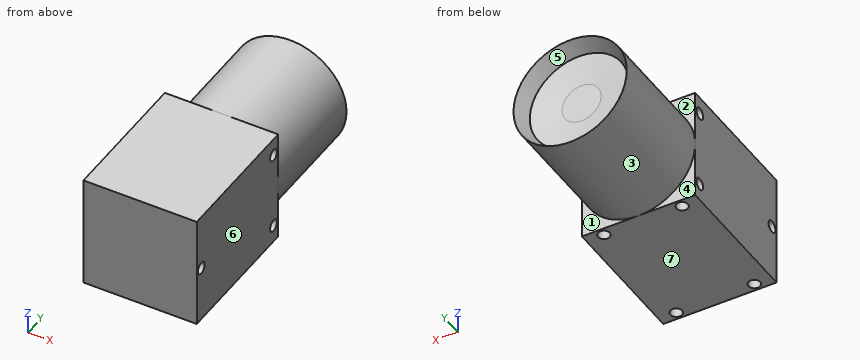
```python
from build123d import *

# Parameters (mm, degrees)
SKETCH_2_W          = 29
SKETCH_2_H          = 29
EXTRUDE_1_DEPTH     = 35.7
SKETCH_3_R          = 1.5
CUT_EXTRUDE_1_DEPTH = 4
CUT_EXTRUDE_2_REACH = 50.226
SKETCH_4_R          = 1.5


with BuildPart() as part:
    # 草图1 → 旋转1 (revolve)
    with BuildSketch(Plane.XY):
        Polygon((0, 0), (-14.5, 0), (-14.5, 30), (-12.646873789, 26.018036841), (-5, 25), (0, 25), align=None)
    revolve(axis=Axis((0, 25, 0), (0, -1, 0)))

    # 草图2 → 凸台-拉伸1 (add)
    with BuildSketch(Plane.XZ):
        Rectangle(SKETCH_2_W, SKETCH_2_H)
    extrude(amount=EXTRUDE_1_DEPTH)

    # 草图3 → 切除-拉伸1 (cut)
    with BuildSketch(Plane(origin=(0, 0, -14.5), x_dir=(-1, 0, 0), z_dir=(0, 0, -1))):
        with Locations((-10, -2)):
            Circle(SKETCH_3_R)
        with Locations((-10, -33.7)):
            Circle(SKETCH_3_R)
        with Locations(Location((10, -33.7, 0), (0, 0, 180))):
            Circle(SKETCH_3_R)
        with Locations(Location((10, -2, 0), (0, 0, 180))):
            Circle(SKETCH_3_R)
    extrude(amount=-CUT_EXTRUDE_1_DEPTH, mode=Mode.SUBTRACT)

    # 草图4 → 切除-拉伸2 (cut, up to next)
    with BuildSketch(Plane(origin=(14.5, 0, 0), x_dir=(0, 0, -1), z_dir=(1, 0, 0)), mode=Mode.PRIVATE) as cut_extrude_2_sk1:
        with Locations(Location((-10, -2, 0), (0, 0, 90))):
            Circle(SKETCH_4_R)
    cut_extrude_2_tool1 = extrude(cut_extrude_2_sk1.sketch, amount=-CUT_EXTRUDE_2_REACH, mode=Mode.PRIVATE) & part.part
    # 草图4 → 切除-拉伸2 (cut, up to next)
    with BuildSketch(Plane(origin=(14.5, 0, 0), x_dir=(0, 0, -1), z_dir=(1, 0, 0)), mode=Mode.PRIVATE) as cut_extrude_2_sk2:
        with Locations(Location((0, -33.7, 0), (0, 0, 90))):
            Circle(SKETCH_4_R)
    cut_extrude_2_tool2 = extrude(cut_extrude_2_sk2.sketch, amount=-CUT_EXTRUDE_2_REACH, mode=Mode.PRIVATE) & part.part
    # 草图4 → 切除-拉伸2 (cut, up to next)
    with BuildSketch(Plane(origin=(14.5, 0, 0), x_dir=(0, 0, -1), z_dir=(1, 0, 0)), mode=Mode.PRIVATE) as cut_extrude_2_sk3:
        with Locations(Location((10, -2, 0), (0, 0, 90))):
            Circle(SKETCH_4_R)
    cut_extrude_2_tool3 = extrude(cut_extrude_2_sk3.sketch, amount=-CUT_EXTRUDE_2_REACH, mode=Mode.PRIVATE) & part.part
    add(cut_extrude_2_tool1.solids().sort_by_distance((14.5, -2, 10))[0], mode=Mode.SUBTRACT)
    add(cut_extrude_2_tool2.solids().sort_by_distance((14.5, -33.7, 0))[0], mode=Mode.SUBTRACT)
    add(cut_extrude_2_tool3.solids().sort_by_distance((14.5, -2, -10))[0], mode=Mode.SUBTRACT)


solid = part.part
```
The listing builds one solid part. Answer for the finished solid, in the listing's coordinates (mm). Face numbers are marked on the shaded views. A direction names the side the tool comes from. Coordinates: 2 decimals unless noted, no trailing zeros. Loops run counter-clockwise (first coordinate to the right, second up) from the corner with the lowest first, then second, coordinate; pieces in that order, holes last. Notation, with made-up numbers: (-22.75, -25) -> (-12.75, -25) arc R8 cw to (-12.75, -11) -> close; hole circle Ø11 at (-15.75, 27). An arc over 180 degrees is marked (long way). Use one line per item in the form item = value. Start each with the question number.
Item 1: Flat-ended cylindrical pins translate along their axes: pin 1 Ø5 at (x, z) = (1, -2) entering from +Y; pin 2 Ø2.5 at (y, z) = (-2, 10) entering from -X; pin 3 Ø11.5 at (x, z) = (5.5, -4) entering from +Y; pin 4 Ø2.5 at (x, y) = (-10, -33.7) entering from -Z. Find the tip coordinate at first contact, or state that the pin passes through.
Item 2: The mould has two halves that part along Z. Classify the marked faces 5, 6 and 7: released by +Z, released by -Z, zero draft, split by the parting line, or undercut.
Item 3: The part is cut by section B-B on x = 2.25. Count the separate pieces of the cut face and the enclosed holes in it, then the cut area to 3 significant figures.
Item 4: A tool of negligible diameter and unlimited length cuts with its end or side. For the marked faces 1, 2, 3 and 4, from which of +Z, -Z, +X, -X, +Y, -Y can it reach the whole face along a straight path? Write none if from no direction.
Item 5: Consider L1, parallel to Z at x = 7, y = -2; L2, parallel to Y at x = -10, z = -13.45; L3, parallel to Y at x = 9.25, z = -12.75. Determine where each line is inside the solid, lowest interval first. Write a range as [from, to].
Item 6: The part is cut by section A-A on y = -33.7. Determine the outline of the cut face in (x, z).
Answer key:
q1.pin_1 = 25
q1.pin_2 = through
q1.pin_3 = 26.01
q1.pin_4 = -10.5
q2.face_5 = undercut
q2.face_6 = zero draft
q2.face_7 = released by -Z
q3.separate_pieces = 1
q3.enclosed_holes = 3
q3.area = 1,750 mm2
q4.face_1 = -Z, +X, +Y
q4.face_2 = +Z, -X, +Y
q4.face_3 = +Y
q4.face_4 = -Z, -X, +Y
q5.L1 = [-14.5, -11.5], [-8.5, 8.5], [11.5, 14.5]
q5.L2 = [-35.7, -35.2], [-32.2, -3.5], [-0.5, 0]
q5.L3 = [-35.7, -35], [-32.4, -3.3], [-0.7, 0]
q6.outline = (-14.5, -14.5) -> (-11.5, -14.5) -> (-11.5, -10.5) -> (-8.5, -10.5) -> (-8.5, -14.5) -> (8.5, -14.5) -> (8.5, -10.5) -> (11.5, -10.5) -> (11.5, -14.5) -> (14.5, -14.5) -> (14.5, -1.5) -> (-14.5, -1.5) -> close; (-14.5, 1.5) -> (14.5, 1.5) -> (14.5, 14.5) -> (-14.5, 14.5) -> close
